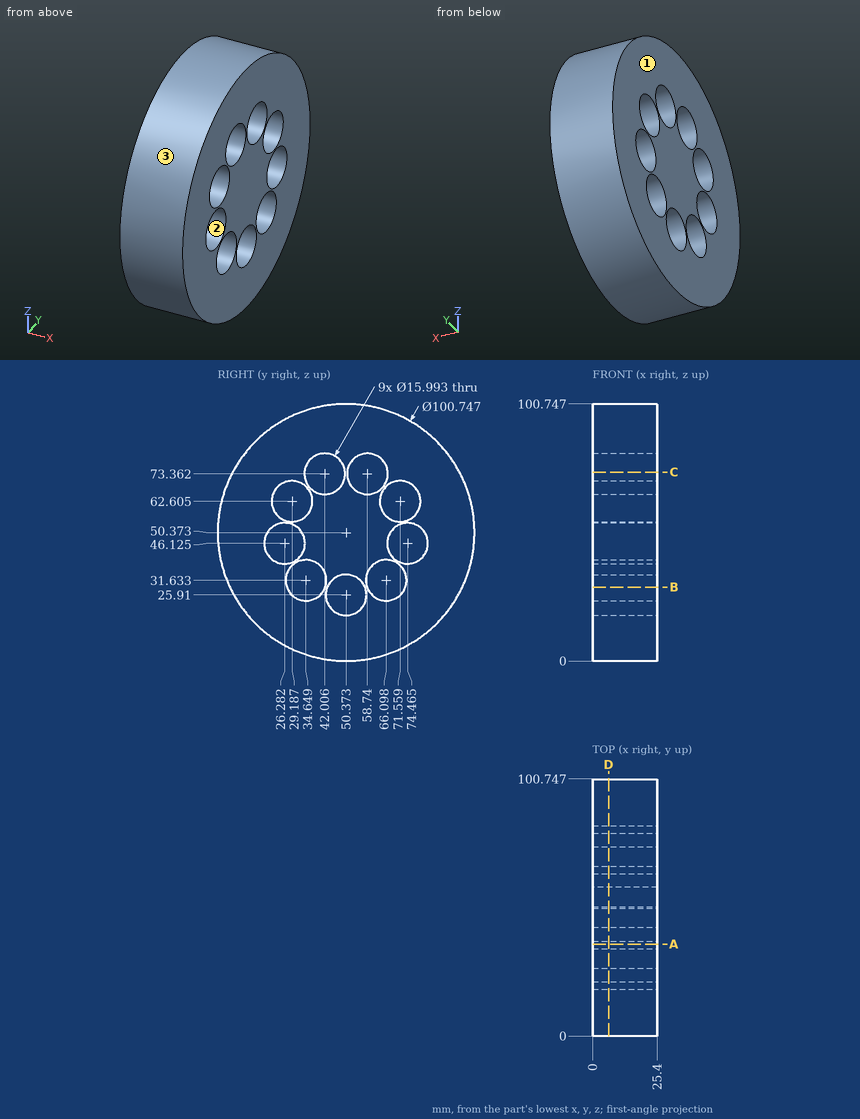
Answer from the drawing. Dimensions are ordinates in mm from the lowest x, y and z of the part. Give positions to 0.01 mm unless a question says otherwise; leave off trailing zeros. Write each loop counter-clockwise with the first axis right and the second up, starting at its lowest first coordinate (ties: lowest second). Pieces come first, ordered by that corner, then holes. Notation, with made-up numbers: (12.25, 88.5) - (22.25, 88.5) arc R26 cw to (22.25, 125.5) - close; hole circle Ø10 at (66.25, 10). An arc over 180 degrees is marked (long way). One line per item, written item: value. Start each with the question number.
1. Consider probe 1 along Y at (x, z) = (11.5, 75) (1 decimal); probe 2 along Y at (x, z) = (11.5, 71) (1 decimal); probe 3 along Z at (x, y) = (17.25, 75) (1 decimal). Determine where each line is inside the solid, lowest interval first.
2. Find section B-B (z = 29). Write down the section's boundary in (x, y).
3. Find section D-D (x = 6.25). State how many separate pieces and enclosed holes the cut face has, then the cut area to 3 significant figures.
4. Find section A-A (y = 36). Write down the section's boundary in (x, z) (1 decimal).
5. Find section C-C (z = 74). Write down the section's boundary in (x, y) (1 decimal).
6. For a pull along Z with two mould halves and no side action, classify the marked faces 1, 2 and 3 as +Z half, -Z half, draft (parallel to the pull), parting line (faces both ways), or undercut.
7. Given pin 1 (5 mm diameter, centred on x = 11.5, z = 12.5, fed in from +Y); pin 2 (9.5 mm diameter, centred on y = 29.19, z = 62.61, fed in from +X); pin 3 (10 mm diameter, centred on x = 22.5, y = 39.5, fed in from +Z); pin 4 (5 mm diameter, centred on x = 10, y = 80.5, fed in from +Z) (1 decimal), each flat-ended and moving along its own axis, determine where each tip first touches the part or whether it passes through.
Geometry results:
1. probe 1: 6.4 to 34.2, 49.8 to 50.9, 66.6 to 94.3
1. probe 2: 4.4 to 34.4, 49.6 to 51.1, 66.4 to 96.3
1. probe 3: 6.4 to 38.1, 54.1 to 55.4, 69.8 to 94.3
2. outline: (0, 4.76) - (25.4, 4.76) - (25.4, 27.1) - (0, 27.1) - close; (0, 42.2) - (25.4, 42.2) - (25.4, 43) - (0, 43) - close; (0, 57.75) - (25.4, 57.75) - (25.4, 58.55) - (0, 58.55) - close; (0, 73.65) - (25.4, 73.65) - (25.4, 95.99) - (0, 95.99) - close
3. separate pieces: 1
3. enclosed holes: 9
3. area: 6,160 mm2
4. outline: (0, 2.1) - (25.4, 2.1) - (25.4, 23.8) - (0, 23.8) - close; (0, 39.5) - (25.4, 39.5) - (25.4, 58.4) - (0, 58.4) - close; (0, 66.8) - (25.4, 66.8) - (25.4, 68.1) - (0, 68.1) - close; (0, 78.6) - (25.4, 78.6) - (25.4, 98.7) - (0, 98.7) - close
5. outline: (0, 5.9) - (25.4, 5.9) - (25.4, 34) - (0, 34) - close; (0, 50) - (25.4, 50) - (25.4, 50.8) - (0, 50.8) - close; (0, 66.7) - (25.4, 66.7) - (25.4, 94.9) - (0, 94.9) - close
6. face 1: draft
6. face 2: undercut
6. face 3: parting line
7. pin 1: y = 86.24
7. pin 2: through
7. pin 3: z = 100.4
7. pin 4: z = 92.5
